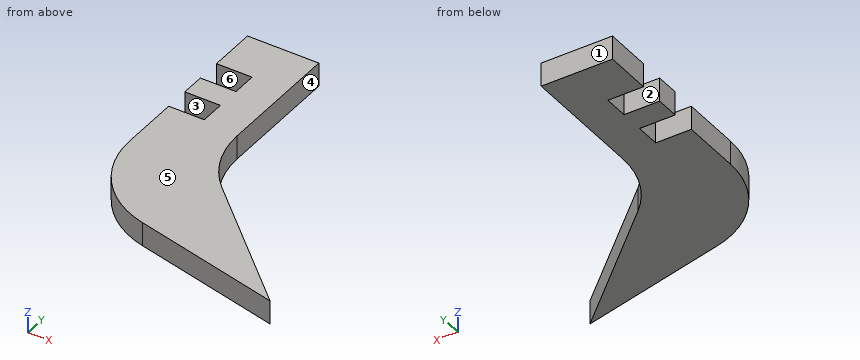
from build123d import *

# Parameters (mm, degrees)
BOSS_EXTRUDE1_DEPTH = 5
FILLET1_R           = 20
FILLET2_R           = 20
SKETCH3_W           = 7.5
SKETCH3_H           = 5.2
CUT_EXTRUDE2_DEPTH  = 5


with BuildPart() as part:
    # Sketch1 → Boss-Extrude1 (new body)
    with BuildSketch(Plane.XY):
        Polygon((0, 53.763883017), (0, 0), (47.193256778, -11.236116983), (15, 18.763883017), (15, 53.763883017), align=None)
    extrude(amount=BOSS_EXTRUDE1_DEPTH)

    # Fillet1
    fillet1_edges = [part.edges().sort_by_distance(p)[0] for p in [
        (0, 0, 2.5),
    ]]
    fillet(fillet1_edges, radius=FILLET1_R)

    # Fillet2
    fillet2_edges = [part.edges().sort_by_distance(p)[0] for p in [
        (15, 18.763883017, 2.5),
    ]]
    fillet(fillet2_edges, radius=FILLET2_R)

    # Sketch3 → Cut-Extrude2 (cut)
    with BuildSketch(Plane.XY):
        with Locations((3.75, 41.163883017)):
            Rectangle(SKETCH3_W, SKETCH3_H)
        with Locations((3.75, 30.963883017)):
            Rectangle(SKETCH3_W, SKETCH3_H)
    extrude(amount=CUT_EXTRUDE2_DEPTH, mode=Mode.SUBTRACT)


solid = part.part
Geometry: final body of the model. Coordinates: model frame, mm. Face numbers are marked on the shaded views. A direction names the side the tool comes from. Give positions to 0.01 mm unless a question says otherwise; leave off trailing zeros. Order: outer loops, then holes, each group sorted by start corner. A loop starts at its lowest first (then second) coordinate and runs counter-clockwise, first axis right, second up. Notation, with made-up numbers: (0, 79.25) -> (52, 79.25) arc R34 ccw to (52, 112.25) -> close; hole circle Ø3 at (38, 45). An arc over 180 degrees is marked (long way). Write each question's results on one line, items separated by ' | '.
1) Set-up query: the marked faces 5 and 6. Return all of +Z, -Z, +X, -X, +Y, -Y with unobstructed straight access to the full face (end or side cutting, diameter ignored); none if empty.
Geometry says:
face 5: +Z, +X, -X, +Y, -Y | face 6: +Z, -Z, -X
2) Draft query along Y for the marked faces 1, 2, 3 and 4. Return one class per face: released by +Y, released by -Y, zero draft, split by the parting line, or undercut.
Geometry says:
face 1: released by +Y | face 2: undercut | face 3: undercut | face 4: zero draft
3) Cut plane A-A (z = 2.1). Output: boundary loops of the cut face in (x, y), and give its area (3 significant figures).
Geometry says:
outline: (0, 15.8) arc R20 ccw to (15.37, -3.66) -> (47.19, -11.24) -> (21.37, 12.83) arc R20 cw to (15, 27.46) -> (15, 53.76) -> (0, 53.76) -> (0, 43.76) -> (7.5, 43.76) -> (7.5, 38.56) -> (0, 38.56) -> (0, 33.56) -> (7.5, 33.56) -> (7.5, 28.36) -> (0, 28.36) -> close | area: 1,080 mm²
4) Cut plane C-C (y = 30). Output: boundary loops of the cut face in (x, z), and give its area (3 significant figures).
Geometry says:
outline: (7.5, 0) -> (15, 0) -> (15, 5) -> (7.5, 5) -> close | area: 37.5 mm²
5) First-contact query: pin 1 Ø2.5 at (x, z) = (4.5, 1.5) entering from -Y; pin 2 Ø1.5 at (y, z) = (45.5, 1.5) entering from +X; pin 3 Ø1.5 at (x, z) = (11, 4.5) entering from -Y. Flat tips, straight axial feed; report the tip coordinate or a pass-through.
Geometry says:
pin 1: stops at y = 1.76 | pin 2: stops at x = 15 | pin 3: stops at y = -2.42
6) Cut plane B-B (x = 4). Output: boundary loops of the cut face in (y, z).
Geometry says:
outline: (3.8, 0) -> (28.36, 0) -> (28.36, 5) -> (3.8, 5) -> close; (33.56, 0) -> (38.56, 0) -> (38.56, 5) -> (33.56, 5) -> close; (43.76, 0) -> (53.76, 0) -> (53.76, 5) -> (43.76, 5) -> close
7) Cut plane D-D (x = 9.5). Output: boundary loops of the cut face in (y, z), and give its area (3 significant figures).
Geometry says:
outline: (-1.22, 0) -> (53.76, 0) -> (53.76, 5) -> (-1.22, 5) -> close | area: 275 mm²
8) Line query: line 1 along Y through (x, z) = (4, 4.75); line 2 along X through (y, z) = (40, 4.2); line 3 along Y through (x, z) = (42, 1). Output: solid intervals per line, ascending.
Geometry says:
line 1: y = 3.8 to 28.36, 33.56 to 38.56, 43.76 to 53.76 | line 2: x = 7.5 to 15 | line 3: y = -10 to -6.4
